The listing builds one solid part. Answer for the finished solid, in the listing's coordinates (mm). A direction names the side the tool comes from. Round coordinates to 2 decimals unless told otherwise and drop trailing zeros. Write each loop counter-clockwise with the first axis right and the second up, starting at its lowest first coordinate (ties: lowest second). Pieces come first, ordered by that corner, then holes.
(1) For faces 4 (the face through (-50.853, 33, 1)), 5 (the face through (-62.99, -47.72, 24.24)), 6 (the face through (-167.853, -31, 1)), determine the directions among +Z, -Z, +X, -X, +Y, -Y from which every point of the face is accessible in a straight line to the end or side of a thin tool.
(2) A cutting plane is placed at C-C, the plane z = -13. Give the vertices of the cut face in (x, y), and give its area (3 significant figures).
(3) A cutting plane is placed at B-B, the plane x = -92. Give the vertices of the cut face in (y, z).
(4) Each of these flat-tipped pins is pushed along its axis until it touches: pin 1 Ø17.5 at (x, z) = (-150.48, -24) entering from +Y; pin 2 Ø6.5 at (x, z) = (-68.48, -24) entering from -Y; pin 3 Ø8 at (y, z) = (10, 34) entering from +X; pin 4 Ø0.9 at (x, z) = (-170, -19.5) entering from +Y. Where does it stop, or does it pass through?
(5) A cutting plane is placed at D-D, the plane z = -32.5. Give the vertices of the cut face in (x, y), and give its area (3 significant figures).
(6) Find the intervals of material crossed by probe 1 along Y at (x, z) = (1, 24.5); probe 2 along Y at (x, z) = (-88.5, 37); probe 3 along X at (y, z) = (87.5, -20), in increasing order.
(7) The mould has two halves that part along Z. Classify faces 1 (the face through (-33, 114, -46)), 2 (the face through (-124, -49.246, 21)), 3 (the face through (-133.33, -47.72, 7.51)): +Z half, -Z half, draft (parallel to the pull), parting line (faces both ways), or undercut.
(8) A cutting plane is placed at A-A, the plane z = 0. Give the vertices of the cut face in (x, y).
from build123d import *

# Parameters (mm, degrees)
F1_DEPTH = 46
F3_D     = 11
F4_D     = 50
F7_D     = 6


# Not quite as in the source:
# - the program builds the solid bodies; features that only make, move or delete a surface that nothing else refers to are left out


with BuildPart() as f1:
    # F0 (on Top) → F1 (new body, symmetric)
    with BuildSketch(Plane.XY):
        with BuildLine():
            Line((-53.8527505398, 110.754218787), (-53.8527505398, -43.245781213))
            ThreePointArc((-53.8527505398, -43.245781213), (-54.7314301962, -45.3671015566), (-56.8527505398, -46.245781213))
            Line((-56.8527505398, -46.245781213), (-164.8527505398, -46.245781213))
            ThreePointArc((-164.8527505398, -46.245781213), (-166.9740708833, -45.3671015566), (-167.8527505398, -43.245781213))
            Line((-167.8527505398, -43.245781213), (-167.8527505398, -19.245781213))
            Line((-167.8527505398, -19.245781213), (-170.8527505398, -19.245781213))
            Line((-170.8527505398, -19.245781213), (-170.8527505398, -43.245781213))
            ThreePointArc((-170.8527505398, -43.245781213), (-169.0953912269, -47.4884219002), (-164.8527505398, -49.245781213))
            Line((-164.8527505398, -49.245781213), (-56.8527505398, -49.245781213))
            ThreePointArc((-56.8527505398, -49.245781213), (-52.6101098527, -47.4884219002), (-50.8527505398, -43.245781213))
            Line((-50.8527505398, -43.245781213), (-50.8527505398, 110.754218787))
            ThreePointArc((-50.8527505398, 110.754218787), (-49.9740708833, 112.8755391305), (-47.8527505398, 113.754218787))
            Line((-47.8527505398, 113.754218787), (21.1472494602, 113.754218787))
            Line((21.1472494602, 113.754218787), (21.1472494602, 116.754218787))
            Line((21.1472494602, 116.754218787), (-47.8527505398, 116.754218787))
            ThreePointArc((-47.8527505398, 116.754218787), (-52.0953912269, 114.9968594741), (-53.8527505398, 110.754218787))
        make_face()
    extrude(amount=F1_DEPTH, both=True)

    # F3 (through all)
    with Locations(Plane.XZ.offset(49.245781213)):
        with Locations((-150.4841212034, 24), (-68.4841212034, 24), (-68.4841212034, -24), (-150.4841212034, -24)):
            Hole(F3_D / 2)

    # F4 (through all)
    with Locations(Plane.XZ.offset(49.245781213)):
        with Locations((-109.4841212034, 0)):
            Hole(F4_D / 2)

    # F7 (through all)
    with Locations(Plane.YZ.offset(-50.8527505398)):
        with Locations((37.5964443088, 0)):
            Hole(F7_D / 2)


solid = f1.part
Solutions:
1. face 4: +Z, -Z, +X, -Y
1. face 5: +Y, -Y
1. face 6: +Z, -Z, +Y
2. outline: (-170.85, -43.25) arc R6 ccw to (-164.85, -49.25) - (-130.84, -49.25) - (-130.84, -46.25) - (-164.85, -46.25) arc R3 cw to (-167.85, -43.25) - (-167.85, -19.25) - (-170.85, -19.25) - close; (-88.13, -49.25) - (-56.85, -49.25) arc R6 ccw to (-50.85, -43.25) - (-50.85, 110.75) arc R3 cw to (-47.85, 113.75) - (21.15, 113.75) - (21.15, 116.75) - (-47.85, 116.75) arc R6 ccw to (-53.85, 110.75) - (-53.85, -43.25) arc R3 cw to (-56.85, -46.25) - (-88.13, -46.25) - close
2. area: 1,000 mm2
3. outline: (-49.25, -46) - (-46.25, -46) - (-46.25, -17.87) - (-49.25, -17.87) - close; (-49.25, 17.87) - (-46.25, 17.87) - (-46.25, 46) - (-49.25, 46) - close
4. pin 1: stops at y = -46.25
4. pin 2: passes through
4. pin 3: stops at x = -50.85
4. pin 4: stops at y = -19.25
5. outline: (-170.85, -43.25) arc R6 ccw to (-164.85, -49.25) - (-56.85, -49.25) arc R6 ccw to (-50.85, -43.25) - (-50.85, 110.75) arc R3 cw to (-47.85, 113.75) - (21.15, 113.75) - (21.15, 116.75) - (-47.85, 116.75) arc R6 ccw to (-53.85, 110.75) - (-53.85, -43.25) arc R3 cw to (-56.85, -46.25) - (-164.85, -46.25) arc R3 cw to (-167.85, -43.25) - (-167.85, -19.25) - (-170.85, -19.25) - close
5. area: 1,130 mm2
6. probe 1: y = 113.75 to 116.75
6. probe 2: y = -49.25 to -46.25
6. probe 3: x = -53.85 to -50.85
7. face 1: -Z half
7. face 2: draft
7. face 3: undercut
8. outline: (-170.85, -43.25) arc R6 ccw to (-164.85, -49.25) - (-134.48, -49.25) - (-134.48, -46.25) - (-164.85, -46.25) arc R3 cw to (-167.85, -43.25) - (-167.85, -19.25) - (-170.85, -19.25) - close; (-84.48, -49.25) - (-56.85, -49.25) arc R6 ccw to (-50.85, -43.25) - (-50.85, 34.6) - (-53.85, 34.6) - (-53.85, -43.25) arc R3 cw to (-56.85, -46.25) - (-84.48, -46.25) - close; (-53.85, 40.6) - (-50.85, 40.6) - (-50.85, 110.75) arc R3 cw to (-47.85, 113.75) - (21.15, 113.75) - (21.15, 116.75) - (-47.85, 116.75) arc R6 ccw to (-53.85, 110.75) - close
